Input: part model. Units: mm. Frame: model coordinates. Face numbers are marked on the shaded views. A direction names the side the tool comes from. Round coordinates to 2 decimals unless told otherwise and drop trailing zeros. Loops run counter-clockwise (first coordinate to the right, second up) from the corner with the lowest first, then second, coordinate; pieces in that order, holes last. Notation, with made-up numbers: (29.5, 66) - (83.5, 66) arc R32 cw to (83.5, 103) - close; hole circle Ø3 at (-23, -32). An arc over 180 degrees is marked (long way). Write each question's results on one line, items separated by ' | '.
from build123d import *

# Parameters (mm, degrees)
FILLET2_R  = 0.6
SKETCH2_W  = 4
SKETCH2_H  = 0.5
SLOT_DEPTH = 0.5


with BuildPart() as part:
    # BodySke → Base-Revolve (revolve)
    with BuildSketch(Plane.XY, mode=Mode.PRIVATE) as base_revolve_sk:
        Polygon((1.3, 1), (1.3, 2), (0, 1.886264737), (0, 0), (21.3, 0), (21.3, 1), align=None)
    revolve(base_revolve_sk.sketch.rotate(Axis((-25.4, 0, 0), (1, 0, 0)), 90), axis=Axis((-25.4, 0, 0), (1, 0, 0)))

    # Fillet2
    fillet2_edges = [part.edges().sort_by_distance(p)[0] for p in [
        (0, 0, -1.886264737),
    ]]
    fillet(fillet2_edges, radius=FILLET2_R)

    # Sketch2 → Slot (cut)
    with BuildSketch(Plane(origin=(0, 0, 0), x_dir=(0, 0, -1), z_dir=(1, 0, 0))):
        Rectangle(SKETCH2_W, SKETCH2_H)
    extrude(amount=SLOT_DEPTH, mode=Mode.SUBTRACT)


solid = part.part
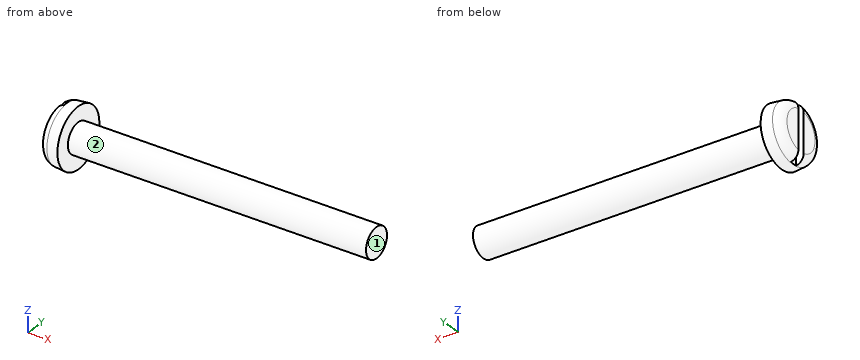
1. Set-up query: the marked faces 1 and 2. Return all of +Z, -Z, +X, -X, +Y, -Y with unobstructed straight access to the full face (end or side cutting, diameter ignored); none if empty.
Answer:
face 1: +Z, -Z, +X, +Y, -Y | face 2: +X
2. Section query B-B, the plane z = 0. Output: boundary loops of the cut face in (x, y).
Answer:
outline: (0, -1.34) arc R0.6 ccw to (0.55, -1.93) - (1.3, -2) - (1.3, -1) - (21.3, -1) - (21.3, 1) - (1.3, 1) - (1.3, 2) - (0.55, 1.93) arc R0.6 ccw to (0, 1.34) - (0, 0.25) - (0.5, 0.25) - (0.5, -0.25) - (0, -0.25) - close
3. Contact query for flat-ended pins moving along their axis: pin 1 (0.6 mm diameter, centred on x = 0, z = -1, fed in from +Y); pin 2 (0.6 mm diameter, centred on x = 0.5, z = 1, fed in from -Y); pin 3 (1 mm diameter, centred on y = 1.5, z = 0.5, fed in from +X). Output: stop coordinate, or through.
Answer:
pin 1: y = 1.62 | pin 2: y = -1.8 | pin 3: x = 1.3
4. Section query C-C, the plane x = 13.5. Output: boundary loops of the cut face in (y, z).
Answer:
outline: circle Ø2 at (0, 0)
5. Line query: line 1 (Y direction, x = 13.75, z = 0); line 2 (X direction, y = -0.5, z = -1.3); line 3 (X direction, y = -0.05, z = -1.55). Output: solid intervals per line, ascending. Write a range as [from, to].
Answer:
line 1: [-1, 1] | line 2: [0, 1.3] | line 3: [0.5, 1.3]
6. Section query A-A, the plane y = 0. Output: boundary loops of the cut face in (x, z), plus the area to 3 significant figures.
Answer:
outline: (0.5, -1.93) arc R0.6 ccw to (0.55, -1.93) - (1.3, -2) - (1.3, -1) - (21.3, -1) - (21.3, 1) - (1.3, 1) - (1.3, 2) - (0.55, 1.93) arc R0.6 ccw to (0.5, 1.93) - close | area: 43.1 mm^2
